For this review, take the finished solid that the model builds, in its own axes (mm). Give positions to 0.01 mm unless a question says otherwise; leave off trailing zeros. Order: outer loops, then holes, each group sorted by start corner. A loop starts at its lowest first (then second) coordinate and runs counter-clockwise, first axis right, second up. Notation, with made-up numbers: M -3,82.25 L 1,82.25 A10 ccw 1,88.25 Z; hole C 23,56 d1. An arc over 180 degrees is marked long. Use CSV: the item, a comma, the result in double quotes. Start each with the question number.
(1) Wall thickness on L1, parallel to X at y = 1.1, z = -21; L2, parallel to Y at x = -8.5, z = 19: over which ranges is each line inside the solid? List them lowest first. Write a range as from..to.
(2) Draft analysis for pull direction Z (two halves, no side actions). For faces 1 (the face through (-1, 1.6, 0)), 2 (the face through (-39, 1.66, 19)), 3 (the face through (-1, 1, 25)), state which applies: pulls with the +Z half, pulls with the -Z half, needs draft (parallel to the pull), parting line crosses it, or undercut.
(3) Consider section A-A (z = -16). Write out the cut boundary in (x, y), and give its area (3 significant figures).
(4) Clearance check with flat-ended pins moving along their axes: P1, Ø6, axis at x = 3.5, z = 12, coming from the -Y side; P2, Ø1, axis at x = 12.5, z = -19, coming from the +Y side. State where each tip first meets the part, or that it passes through.
(5) Consider section B-B (x = 28.5). Write out the cut boundary in (y, z), and give its area (3 significant figures).
```python
from build123d import *

# Parameters (mm, degrees)
SKETCH_1_W          = 86
SKETCH_1_H          = 50
EXTRUDE_1_DEPTH     = 1.6
SKETCH_2_R          = 2.8
SKETCH_2_R_2        = 1.6
EXTRUDE_2_DEPTH     = 0.06
SKETCH_4_R          = 1.6
CUT_EXTRUDE_1_DEPTH = 50.765047975
FILLET_1_R          = 3.5


with BuildPart() as part:
    # 草图1 → 凸台-拉伸1 (new body)
    with BuildSketch(Plane(origin=(0, 0, 0), x_dir=(1, 0, 0), z_dir=(0, 1, 0))):
        Rectangle(SKETCH_1_W, SKETCH_1_H)
    extrude(amount=EXTRUDE_1_DEPTH)

    # 草图2 → 凸台-拉伸2 (add)
    # profile 1 of 4: a face of its own
    with BuildSketch(Plane(origin=(0, 1.6, 0), x_dir=(1, 0, 0), z_dir=(0, 1, 0))):
        with Locations(Location((-39, 21, 0), (0, 0, 90))):
            Circle(SKETCH_2_R)
        with Locations(Location((-39, 21, 0), (0, 0, 270))):
            Circle(SKETCH_2_R_2, mode=Mode.SUBTRACT)
    # profile 2 of 4: a face of its own
    with BuildSketch(Plane(origin=(0, 1.6, 0), x_dir=(1, 0, 0), z_dir=(0, 1, 0))):
        with Locations(Location((39, 21, 0), (0, 0, 90))):
            Circle(SKETCH_2_R)
        with Locations(Location((39, 21, 0), (0, 0, 270))):
            Circle(SKETCH_2_R_2, mode=Mode.SUBTRACT)
    # profile 3 of 4: a face of its own
    with BuildSketch(Plane(origin=(0, 1.6, 0), x_dir=(1, 0, 0), z_dir=(0, 1, 0))):
        with Locations(Location((39, -21, 0), (0, 0, 90))):
            Circle(SKETCH_2_R)
        with Locations(Location((39, -21, 0), (0, 0, 270))):
            Circle(SKETCH_2_R_2, mode=Mode.SUBTRACT)
    # profile 4 of 4: a face of its own
    with BuildSketch(Plane(origin=(0, 1.6, 0), x_dir=(1, 0, 0), z_dir=(0, 1, 0))):
        with Locations(Location((-39, -21, 0), (0, 0, 90))):
            Circle(SKETCH_2_R)
        with Locations(Location((-39, -21, 0), (0, 0, 270))):
            Circle(SKETCH_2_R_2, mode=Mode.SUBTRACT)
    extrude(amount=EXTRUDE_2_DEPTH)

    # 草图4 → 切除-拉伸1 (cut, through all)
    with BuildSketch(Plane(origin=(0, 1.6, 0), x_dir=(1, 0, 0), z_dir=(0, 1, 0))):
        with Locations(Location((-39, 21, 0), (0, 0, 270))):
            Circle(SKETCH_4_R)
        with Locations(Location((39, 21, 0), (0, 0, 270))):
            Circle(SKETCH_4_R)
        with Locations(Location((39, -21, 0), (0, 0, 270))):
            Circle(SKETCH_4_R)
        with Locations(Location((-39, -21, 0), (0, 0, 270))):
            Circle(SKETCH_4_R)
    extrude(amount=-CUT_EXTRUDE_1_DEPTH, mode=Mode.SUBTRACT)

    # 圆角1
    fillet_1_edges = [part.edges().sort_by_distance(p)[0] for p in [
        (43, 0.8, 25),
        (-43, 0.8, 25),
        (-43, 0.8, -25),
        (43, 0.8, -25),
    ]]
    fillet(fillet_1_edges, radius=FILLET_1_R)


solid = part.part
```
Check result:
1,L1,"x = -43..-40.6, -37.4..37.4, 40.6..43"
1,L2,"y = 0..1.6"
2,face 1,"undercut"
2,face 2,"needs draft"
2,face 3,"pulls with the +Z half"
3,outline,"M -43,0 L 43,0 L 43,1.6 L -43,1.6 Z"
3,area,"138 mm^2"
4,P1,"stops at y = 0"
4,P2,"stops at y = 1.6"
5,outline,"M 0,-25 L 1.6,-25 L 1.6,25 L 0,25 Z"
5,area,"80.0 mm^2"
